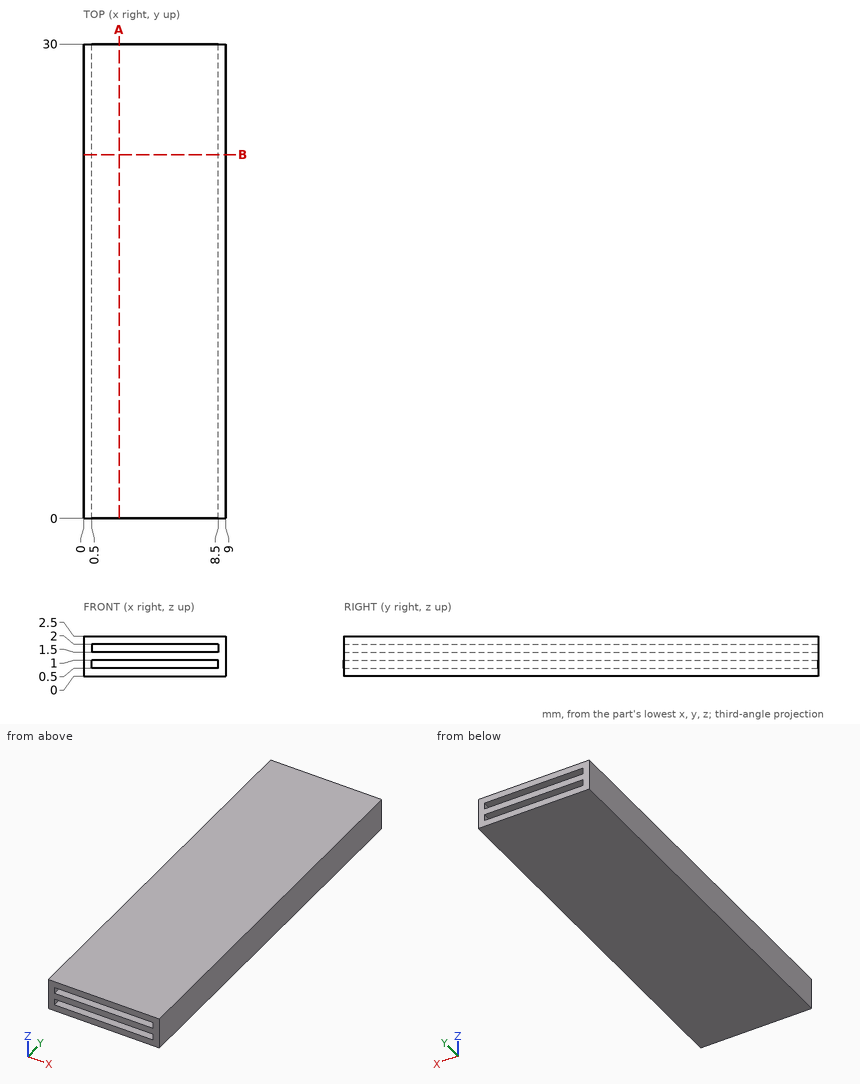
Answer from the drawing. Dimensions are ordinates in mm from the lowest x, y and z of the part. Round coordinates to 2 decimals unless told otherwise and drop trailing zeros. Write each loop counter-clockwise with the first axis right and the second up, starting at its lowest first coordinate (ties: lowest second). Pieces come first, ordered by that corner, then holes.
1. Straight lines are drawn through the part: L1, parallel to Z at x = 3, y = 21.75; L2, parallel to X at y = 9.5, z = 0.9. For each, find the intervals that lie inside material, in ascending order.
2. Given pin 1 Ø2 at (x, y) = (2.5, 13.5) entering from -Z, flat-ended and moving along its own axis, determine where the tip first touches the part or whether it passes through.
3. The part is cut by section A-A, the plane x = 2.25. Determine the outline of the cut face in (y, z).
4. The part is cut by section B-B, the plane y = 23. Determine the outline of the cut face in (x, z).
Values:
1. L1: z = 0 to 0.5, 1 to 1.5, 2 to 2.5
1. L2: x = 0 to 0.5, 8.5 to 9
2. pin 1: stops at z = 0
3. outline: (0, 0) - (30, 0) - (30, 0.5) - (0, 0.5) - close; (0, 1) - (30, 1) - (30, 1.5) - (0, 1.5) - close; (0, 2) - (30, 2) - (30, 2.5) - (0, 2.5) - close
4. outline: (0, 0) - (9, 0) - (9, 2.5) - (0, 2.5) - close; hole (0.5, 0.5) - (8.5, 0.5) - (8.5, 1) - (0.5, 1) - close; hole (0.5, 1.5) - (8.5, 1.5) - (8.5, 2) - (0.5, 2) - close
